from build123d import *

# Parameters (mm, degrees)
BOSS_EXTRUDE1_DEPTH       = 16
F_1_0MM_DOWEL_HOLE1_D     = 20
F_1_0MM_DOWEL_HOLE1_DEPTH = 26.4
F_1_0MM_DOWEL_HOLE1_TIP   = 6.00860619


with BuildPart() as part:
    # Sketch1 → Boss-Extrude1 (new body)
    with BuildSketch(Plane(origin=(0, 0, 0), x_dir=(1, 0, 0), z_dir=(0, 1, 0))):
        Polygon((19.975, 0), (9.9875, 17.298857441), (-9.9875, 17.298857441), (-19.975, 0), (-9.9875, -17.298857441), (9.9875, -17.298857441), align=None)
    extrude(amount=BOSS_EXTRUDE1_DEPTH)

    # Sketch2 → Revolve1 (revolve)
    with BuildSketch(Plane.ZY):
        with BuildLine():
            Line((-17.298857441, 16), (-17.298857441, 16.101142559))
            ThreePointArc((-17.298857441, 16.101142559), (-12.232139403, 28.333281962), (0, 33.4))
            Line((0, 33.4), (0, 16))
            Line((0, 16), (-17.298857441, 16))
        make_face()
    revolve(axis=Axis((0, 16, 0), (0, 1, 0)))

    # Ø1.0mm Dowel Hole1
    with Locations(Plane(origin=(0, 0, 0), x_dir=(-1, 0, 0), z_dir=(0, -1, 0))):
        with Locations((0, 0)):
            Hole(F_1_0MM_DOWEL_HOLE1_D / 2, depth=F_1_0MM_DOWEL_HOLE1_DEPTH)
            with Locations((0, 0, -(F_1_0MM_DOWEL_HOLE1_DEPTH + F_1_0MM_DOWEL_HOLE1_TIP / 2))):  # 118° drill point
                Cone(0, F_1_0MM_DOWEL_HOLE1_D / 2, F_1_0MM_DOWEL_HOLE1_TIP, mode=Mode.SUBTRACT)

    # Sketch6 → Cut-Revolve1 (revolve, cut)
    with BuildSketch(Plane.XY, mode=Mode.PRIVATE) as cut_revolve1_sk:
        Polygon((17.298857441, 16), (19.975, 13.323857441), (19.975, 16), align=None)
        Polygon((19.975, 2.676142559), (19.975, 0), (17.298857441, 0), align=None)
    revolve(cut_revolve1_sk.sketch.rotate(Axis((0, 16, 0), (0, 1, 0)), 90), axis=Axis((0, 16, 0), (0, 1, 0)), mode=Mode.SUBTRACT)


solid = part.part
The listing builds one solid part. Answer for the finished solid, in the listing's coordinates (mm). Coordinates: 2 decimals unless noted, no trailing zeros. Loops run counter-clockwise (first coordinate to the right, second up) from the corner with the lowest first, then second, coordinate; pieces in that order, holes last. Notation, with made-up numbers: (58, 71) -> (112, 71) arc R16 cw to (112, 83) -> close; hole circle Ø4 at (71, 74). An arc over 180 degrees is marked (long way). Answer in a Markdown table with one row per item. Add a question column.
1. The part is cut by section A-A, the plane y = 9. Write down the section's boundary in (x, z) (1 decimal), then the cut area to 3 significant figures.
2. Flat-ended cylindrical pins translate along their axes: P1, Ø1, axis at y = 21, z = -10, coming from the +X side; P2, Ø1.5, axis at x = 13, y = 11.5, coming from the -Z side; P3, Ø6, axis at y = 4.5, z = 7.5, coming from the -X side. Find the tip coordinate at first contact, or state that the pin passes through.
3. The part is cut by section B-B, the plane y = 23. Write down the section's boundary in (x, z), then the cut area to 3 significant figures.
4. Consider line 1 (Y direction, x = -8.5, z = -11); line 2 (X direction, y = 2, z = 6); line 3 (X direction, y = 2.5, z = -3). Determine where each line is inside the solid, lowest interval first. Write a range as [from, to].
5. Determine the mould class of faces 1 (the conical face through (-8.937, 15.349, -15.566)), 2 (the flat face through (-15.05, 7.89, 8.53)), 3 (the conical face through (0.376, 31.365, 1.695)) for opening direction Z: +Z half, -Z half, draft (parallel to the pull), parting line (faces both ways), or undercut.
Answer below:
| question | item | result |
|---|---|---|
| 1 | outline | (-20, 0) -> (-10, -17.3) -> (10, -17.3) -> (20, 0) -> (10, 17.3) -> (-10, 17.3) -> close; hole circle Ø20 at (0, 0) |
| 1 | area | 722 mm2 |
| 2 | P1 | x = 13.64 |
| 2 | P2 | z = -13.38 |
| 2 | P3 | x = -17.38 |
| 3 | outline | circle Ø31.73 at (0, 0); hole circle Ø20 at (0, 0) |
| 3 | area | 476 mm2 |
| 4 | line 1 | [0, 26.4] |
| 4 | line 2 | [-16.51, -8], [8, 16.51] |
| 4 | line 3 | [-18.24, -9.54], [9.54, 18.24] |
| 5 | face 1 | -Z half |
| 5 | face 2 | +Z half |
| 5 | face 3 | undercut |
